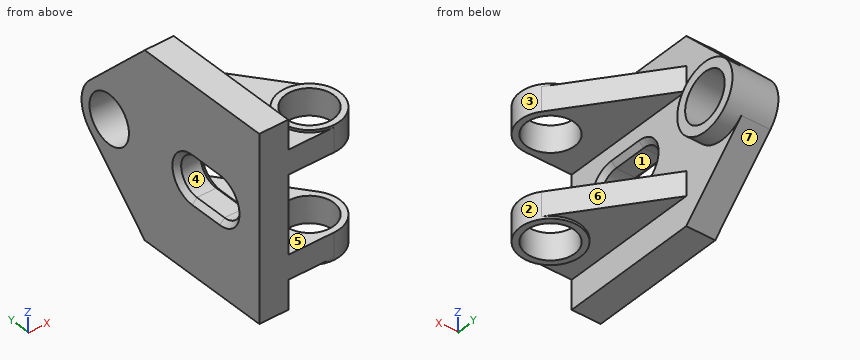
```python
from build123d import *

# Parameters (mm, degrees)
BOSS_EXTRUDE1_DEPTH = 12
SKETCH1_3_R         = 14
SKETCH1_3_R_2       = 10
BOSS_EXTRUDE2_DEPTH = 19
BOSS_EXTRUDE3_START = 16
BOSS_EXTRUDE3_DEPTH = 10
BOSS_EXTRUDE4_START = 16
SKETCH2_4_R         = 12.5
SKETCH2_4_R_2       = 10
BOSS_EXTRUDE4_DEPTH = 11
CHAMFER1_SIZE       = 2


with BuildPart() as part:
    # Sketch1 → Boss-Extrude1 (new body)
    with BuildSketch(Plane(origin=(0, 0, 0), x_dir=(0, 0, -1), z_dir=(1, 0, 0))):
        with BuildLine():
            Line((38, 0), (38, 58))
            Line((38, 58), (9.863920086, 85.934942403))
            ThreePointArc((9.863920086, 85.934942403), (12.924683385, 81.380758255), (14, 76))
            ThreePointArc((14, 76), (-5.380758255, 63.075316615), (-9.863920086, 85.934942403))
            Line((-9.863920086, 85.934942403), (-38, 58))
            Line((-38, 58), (-38, 0))
            Line((-38, 0), (38, 0))
        make_face()
        with BuildLine():
            ThreePointArc((-8, 34), (0, 42), (8, 34))
            Line((8, 34), (8, 20))
            ThreePointArc((8, 20), (0, 12), (-8, 20))
            Line((-8, 20), (-8, 34))
        make_face(mode=Mode.SUBTRACT)
    extrude(amount=BOSS_EXTRUDE1_DEPTH)

    # Sketch1_3 → Boss-Extrude2 (add)
    with BuildSketch(Plane(origin=(0, 0, 0), x_dir=(0, 0, -1), z_dir=(1, 0, 0))):
        with Locations(Location((0, 76, 0), (0, 0, 134.794469931))):
            Circle(SKETCH1_3_R)
        with Locations((0, 76)):
            Circle(SKETCH1_3_R_2, mode=Mode.SUBTRACT)
    extrude(amount=BOSS_EXTRUDE2_DEPTH)

    # Sketch2 → Boss-Extrude3 (add)
    with BuildSketch(Plane.XY.offset(BOSS_EXTRUDE3_START)):
        with BuildLine():
            Line((12, 58), (12, 0))
            Line((12, 0), (31, 0))
            ThreePointArc((31, 0), (19.796343324, 18.043291177), (40.936820993, 20.083507668))
            Line((40.936820993, 20.083507668), (12, 58))
        make_face()
    boss_extrude3 = extrude(amount=BOSS_EXTRUDE3_DEPTH)

    # Sketch2_4 → Boss-Extrude4 (add)
    with BuildSketch(Plane.XY.offset(BOSS_EXTRUDE4_START)):
        with Locations(Location((31, 12.5, 0), (0, 0, 270))):
            Circle(SKETCH2_4_R)
        with Locations((31, 12.5)):
            Circle(SKETCH2_4_R_2, mode=Mode.SUBTRACT)
    boss_extrude4 = extrude(amount=BOSS_EXTRUDE4_DEPTH)

    # Mirror2: Boss-Extrude3, Boss-Extrude4 across plane
    add(boss_extrude3.mirror(Plane.XY))
    add(boss_extrude4.mirror(Plane.XY))

    # Chamfer1
    chamfer1_edges = [part.edges().sort_by_distance(p)[0] for p in [
        (12, 27, 8),
        (0, 27, -8),
        (0, 42, 0),
        (0, 27, 8),
        (0, 12, 0),
        (12, 42, 0),
        (12, 27, -8),
        (12, 12, 0),
    ]]
    chamfer(chamfer1_edges, length=CHAMFER1_SIZE)


solid = part.part
```
Geometry: final body of the model. Coordinates: model frame, mm. Face numbers are marked on the shaded views. A direction names the side the tool comes from. Round coordinates to 2 decimals unless told otherwise and drop trailing zeros. Loops run counter-clockwise (first coordinate to the right, second up) from the corner with the lowest first, then second, coordinate; pieces in that order, holes last. Notation, with made-up numbers: (43.25, 57) -> (85.25, 57) arc R22 cw to (85.25, 86) -> close; hole circle Ø4 at (7.5, 3.5). An arc over 180 degrees is marked (long way). Write each question's results on one line, items separated by ' | '.
Item 1: Cut plane A-A on z = 0. Return the cut outline in (x, y), and give its area (3 significant figures).
Answers below:
outline: (0, 0) -> (12, 0) -> (12, 10) -> (10, 12) -> (2, 12) -> (0, 10) -> close; (0, 44) -> (2, 42) -> (10, 42) -> (12, 44) -> (12, 62) -> (19, 62) -> (19, 66) -> (0, 66) -> close; (0, 86) -> (19, 86) -> (19, 90) -> (0, 90) -> close | area: 528 mm²
Item 2: Line query: probe 1 along X at (y, z) = (12, -23); probe 2 along Y at (x, z) = (6, 6); probe 3 along Y at (x, z) = (14.75, 0). Output: solid intervals per line, ascending. Write a range as [from, to].
Answers below:
probe 1: x = [0, 21.01], [40.99, 43.49] | probe 2: y = [0, 14.71], [39.29, 68], [84, 88.65] | probe 3: y = [62, 66], [86, 90]
Item 3: Set-up query: the marked faces 1, 2 and 3. Return all of +Z, -Z, +X, -X, +Y, -Y with unobstructed straight access to the full face (end or side cutting, diameter ignored); none if empty.
Answers below:
face 1: +X, -X | face 2: -Z | face 3: +Z
Item 4: Cut plane B-B on x = 34. Return the cut outline in (y, z).
Answers below:
outline: (0.37, -27) -> (2.96, -27) -> (2.96, -16) -> (0.37, -16) -> close; (0.37, 16) -> (2.96, 16) -> (2.96, 27) -> (0.37, 27) -> close; (22.04, -27) -> (24.63, -27) -> (24.63, -26) -> (29.17, -26) -> (29.17, -16) -> (22.04, -16) -> close; (22.04, 16) -> (29.17, 16) -> (29.17, 26) -> (24.63, 26) -> (24.63, 27) -> (22.04, 27) -> close
Item 5: Pull-direction query (Z, two-part tool) for the marked faces 4, 5, 6 and 7; classes: pulls with the +Z half, pulls with the -Z half, needs draft (parallel to the pull), parting line crosses it, or undercut.
Answers below:
face 4: undercut | face 5: undercut | face 6: needs draft | face 7: pulls with the -Z half
Item 6: Cut plane C-C on x = 15. Return the cut outline in (y, z).
Answers below:
outline: (0, -26) -> (54.07, -26) -> (54.07, -16) -> (0, -16) -> close; (0, 16) -> (54.07, 16) -> (54.07, 26) -> (0, 26) -> close; circle Ø28 at (76, 0); hole circle Ø20 at (76, 0)
Item 7: Pin query (flat end, axial travel): pin 1 Ø6 at (y, z) = (69.5, -24.5) entering from +X; pin 2 Ø20 at (x, y) = (37, 17) entering from +Z; pin 3 Ø12.5 at (x, y) = (30.5, 7.5) entering from -Z. Return the tip coordinate at first contact, or that it passes through.
Answers below:
pin 1: stops at x = 12 | pin 2: stops at z = 27 | pin 3: stops at z = -27
Item 8: Cut plane D-D on y = 76. Return the cut outline in (x, z), and give its area (3 significant figures).
Answers below:
outline: (0, -19.87) -> (12, -19.87) -> (12, -14) -> (19, -14) -> (19, -10) -> (0, -10) -> close; (0, 10) -> (19, 10) -> (19, 14) -> (12, 14) -> (12, 19.87) -> (0, 19.87) -> close | area: 293 mm²
